For this review, use the dimensioned drawing (mm, ordinates from the lowest corner) and the shaded views. Give positions to 0.01 mm unless a question says otherwise; leave off trailing zeros. Write each loop counter-clockwise with the first axis right and the second up, starting at its lowest first coordinate (ties: lowest second). Pieces come first, ordered by that corner, then holes. Notation, with made-up numbers: (-2.5, 5) -> (30.5, 5) arc R25 ccw to (30.5, 38) -> close; hole circle Ø7 at (33, 0.5). An arc over 180 degrees is marked (long way). Answer as CSV lines item,"result".
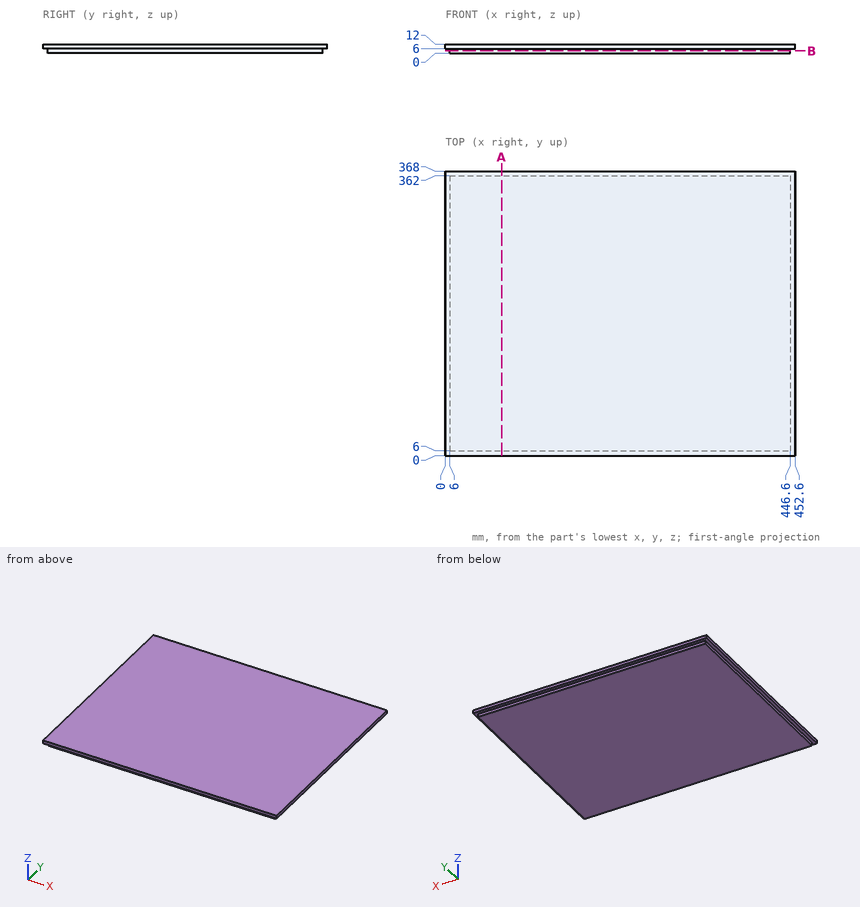
Q1. Add section A-A (x = 73). Write out the cut boundary in (y, z), plus the area to 3 significant figures.
Answer block:
outline,"(0, 6) -> (6, 6) -> (6, 0) -> (362, 0) -> (362, 6) -> (368, 6) -> (368, 12) -> (0, 12) -> close"
area,"4,340 mm2"
Q2. To check wall thickness, follow probe 1 along Y at (x, z) = (166.5, 2); probe 2 along X at (y, z) = (51.5, 2). State the ranges of each line that lie inside material, in increasing order. Write a range as [from, to].
Answer block:
probe 1,"y = [6, 362]"
probe 2,"x = [6, 446.6]"
Q3. Add section B-B (z = 3.25). Write out the cut boundary in (x, y), plus the area to 3 significant figures.
Answer block:
outline,"(6, 6) -> (446.6, 6) -> (446.6, 362) -> (6, 362) -> close"
area,"157,000 mm2"
Q4. Clearance check with flat-ended pins moving along their axes: pin 1 (5 mm diameter, centred on x = 279, z = 3, fed in from +Y); pin 2 (5 mm diameter, centred on x = 188, z = 1.5, fed in from -Y); pin 3 (3 mm diameter, centred on y = 261, z = 3.5, fed in from +X). State where each tip first meets the part, or that it passes through.
Answer block:
pin 1,"stops at y = 362"
pin 2,"stops at y = 6"
pin 3,"stops at x = 446.6"
